Work out the finished part from the listing and answer in its coordinate system (mm). Face numbers are marked on the shaded views. Round coordinates to 2 decimals unless told otherwise and drop trailing zeros. One line per item, written item: value.
```python
from build123d import *

# Parameters (mm, degrees)
CELL_BLOCK_SKETCH_W  = 140.101132068
CELL_BLOCK_SKETCH_H  = 360.075
BOSS_EXTRUDE1_DEPTH  = 5
CELL_HOLES_PATTERN_R = 10.875
CUT_EXTRUDE1_DEPTH   = 5
SKETCH1_R            = 10.875
CUT_EXTRUDE2_DEPTH   = 5
SKETCH3_W            = 15
SKETCH3_H            = 360.075
BOSS_EXTRUDE3_DEPTH  = 10
SKETCH4_R            = 3.25
CUT_EXTRUDE3_DEPTH   = 10


with BuildPart() as part:
    # Cell Block Sketch → Boss-Extrude1 (new body)
    with BuildSketch(Plane(origin=(0, 0, 0), x_dir=(1, 0, 0), z_dir=(0, 1, 0))):
        Rectangle(CELL_BLOCK_SKETCH_W, CELL_BLOCK_SKETCH_H)
    extrude(amount=BOSS_EXTRUDE1_DEPTH)

    # Cell Holes Pattern → Cut-Extrude1 (cut)
    with BuildSketch(Plane(origin=(0, 0, 0), x_dir=(1, 0, 0), z_dir=(0, 1, 0))):
        with Locations(Location((-34.400283017, 137.7875, 0), (0, 0, 270))):
            Circle(CELL_HOLES_PATTERN_R)
        with Locations(Location((-54.275566034, 149.2625, 0), (0, 0, 270))):
            Circle(CELL_HOLES_PATTERN_R)
        with Locations(Location((-14.525, 149.2625, 0), (0, 0, 270))):
            Circle(CELL_HOLES_PATTERN_R)
        with Locations(Location((-54.275566034, 126.3125, 0), (0, 0, 270))):
            Circle(CELL_HOLES_PATTERN_R)
        with Locations(Location((-34.400283017, 114.8375, 0), (0, 0, 270))):
            Circle(CELL_HOLES_PATTERN_R)
        with Locations(Location((-14.525, 126.3125, 0), (0, 0, 270))):
            Circle(CELL_HOLES_PATTERN_R)
        with Locations(Location((-54.275566034, 103.3625, 0), (0, 0, 270))):
            Circle(CELL_HOLES_PATTERN_R)
        with Locations(Location((-34.400283017, 91.8875, 0), (0, 0, 270))):
            Circle(CELL_HOLES_PATTERN_R)
        with Locations(Location((-14.525, 103.3625, 0), (0, 0, 270))):
            Circle(CELL_HOLES_PATTERN_R)
        with Locations(Location((-54.275566034, 80.4125, 0), (0, 0, 270))):
            Circle(CELL_HOLES_PATTERN_R)
        with Locations(Location((-34.400283017, 68.9375, 0), (0, 0, 270))):
            Circle(CELL_HOLES_PATTERN_R)
        with Locations(Location((-14.525, 80.4125, 0), (0, 0, 270))):
            Circle(CELL_HOLES_PATTERN_R)
        with Locations(Location((-54.275566034, 57.4625, 0), (0, 0, 270))):
            Circle(CELL_HOLES_PATTERN_R)
        with Locations(Location((-34.400283017, 45.9875, 0), (0, 0, 270))):
            Circle(CELL_HOLES_PATTERN_R)
        with Locations(Location((-14.525, 57.4625, 0), (0, 0, 270))):
            Circle(CELL_HOLES_PATTERN_R)
        with Locations(Location((-54.275566034, 34.5125, 0), (0, 0, 270))):
            Circle(CELL_HOLES_PATTERN_R)
        with Locations(Location((-34.400283017, 23.0375, 0), (0, 0, 270))):
            Circle(CELL_HOLES_PATTERN_R)
        with Locations(Location((-14.525, 34.5125, 0), (0, 0, 270))):
            Circle(CELL_HOLES_PATTERN_R)
        with Locations(Location((-54.275566034, 11.5625, 0), (0, 0, 270))):
            Circle(CELL_HOLES_PATTERN_R)
        with Locations(Location((-34.400283017, 0.0875, 0), (0, 0, 270))):
            Circle(CELL_HOLES_PATTERN_R)
        with Locations(Location((-14.525, 11.5625, 0), (0, 0, 270))):
            Circle(CELL_HOLES_PATTERN_R)
        with Locations(Location((-54.275566034, -11.3875, 0), (0, 0, 270))):
            Circle(CELL_HOLES_PATTERN_R)
        with Locations(Location((-34.400283017, -22.8625, 0), (0, 0, 270))):
            Circle(CELL_HOLES_PATTERN_R)
        with Locations(Location((-14.525, -11.3875, 0), (0, 0, 270))):
            Circle(CELL_HOLES_PATTERN_R)
        with Locations(Location((-54.275566034, -34.3375, 0), (0, 0, 270))):
            Circle(CELL_HOLES_PATTERN_R)
        with Locations(Location((-34.400283017, -45.8125, 0), (0, 0, 270))):
            Circle(CELL_HOLES_PATTERN_R)
        with Locations(Location((-14.525, -34.3375, 0), (0, 0, 270))):
            Circle(CELL_HOLES_PATTERN_R)
        with Locations(Location((-54.275566034, -57.2875, 0), (0, 0, 270))):
            Circle(CELL_HOLES_PATTERN_R)
        with Locations(Location((-34.400283017, -68.7625, 0), (0, 0, 270))):
            Circle(CELL_HOLES_PATTERN_R)
        with Locations(Location((-14.525, -57.2875, 0), (0, 0, 270))):
            Circle(CELL_HOLES_PATTERN_R)
        with Locations(Location((-54.275566034, -80.2375, 0), (0, 0, 270))):
            Circle(CELL_HOLES_PATTERN_R)
        with Locations(Location((-34.400283017, -91.7125, 0), (0, 0, 270))):
            Circle(CELL_HOLES_PATTERN_R)
        with Locations(Location((-14.525, -80.2375, 0), (0, 0, 270))):
            Circle(CELL_HOLES_PATTERN_R)
        with Locations(Location((-54.275566034, -103.1875, 0), (0, 0, 270))):
            Circle(CELL_HOLES_PATTERN_R)
        with Locations(Location((-34.400283017, -114.6625, 0), (0, 0, 270))):
            Circle(CELL_HOLES_PATTERN_R)
        with Locations(Location((-14.525, -103.1875, 0), (0, 0, 270))):
            Circle(CELL_HOLES_PATTERN_R)
        with Locations(Location((-54.275566034, -126.1375, 0), (0, 0, 270))):
            Circle(CELL_HOLES_PATTERN_R)
        with Locations(Location((-34.400283017, -137.6125, 0), (0, 0, 270))):
            Circle(CELL_HOLES_PATTERN_R)
        with Locations(Location((-14.525, -126.1375, 0), (0, 0, 270))):
            Circle(CELL_HOLES_PATTERN_R)
        with Locations(Location((-54.275566034, -149.0875, 0), (0, 0, 270))):
            Circle(CELL_HOLES_PATTERN_R)
        with Locations(Location((-34.400283017, -160.5625, 0), (0, 0, 270))):
            Circle(CELL_HOLES_PATTERN_R)
        with Locations(Location((-14.525, -149.0875, 0), (0, 0, 270))):
            Circle(CELL_HOLES_PATTERN_R)
    extrude(amount=CUT_EXTRUDE1_DEPTH, mode=Mode.SUBTRACT)

    # Sketch1 → Cut-Extrude2 (cut)
    with BuildSketch(Plane(origin=(0, 5, 0), x_dir=(1, 0, 0), z_dir=(0, 1, 0))):
        with Locations(Location((14.525, 137.7875, 0), (0, 0, 270))):
            Circle(SKETCH1_R)
        with Locations(Location((34.400283017, 149.2625, 0), (0, 0, 270))):
            Circle(SKETCH1_R)
        with Locations(Location((54.275566034, 137.7875, 0), (0, 0, 270))):
            Circle(SKETCH1_R)
        with Locations(Location((14.525, 114.8375, 0), (0, 0, 270))):
            Circle(SKETCH1_R)
        with Locations(Location((34.400283017, 126.3125, 0), (0, 0, 270))):
            Circle(SKETCH1_R)
        with Locations(Location((54.275566034, 114.8375, 0), (0, 0, 270))):
            Circle(SKETCH1_R)
        with Locations(Location((14.525, 91.8875, 0), (0, 0, 270))):
            Circle(SKETCH1_R)
        with Locations(Location((34.400283017, 103.3625, 0), (0, 0, 270))):
            Circle(SKETCH1_R)
        with Locations(Location((54.275566034, 91.8875, 0), (0, 0, 270))):
            Circle(SKETCH1_R)
        with Locations(Location((14.525, 68.9375, 0), (0, 0, 270))):
            Circle(SKETCH1_R)
        with Locations(Location((34.400283017, 80.4125, 0), (0, 0, 270))):
            Circle(SKETCH1_R)
        with Locations(Location((54.275566034, 68.9375, 0), (0, 0, 270))):
            Circle(SKETCH1_R)
        with Locations(Location((14.525, 45.9875, 0), (0, 0, 270))):
            Circle(SKETCH1_R)
        with Locations(Location((34.400283017, 57.4625, 0), (0, 0, 270))):
            Circle(SKETCH1_R)
        with Locations(Location((54.275566034, 45.9875, 0), (0, 0, 270))):
            Circle(SKETCH1_R)
        with Locations(Location((14.525, 23.0375, 0), (0, 0, 270))):
            Circle(SKETCH1_R)
        with Locations(Location((34.400283017, 34.5125, 0), (0, 0, 270))):
            Circle(SKETCH1_R)
        with Locations(Location((54.275566034, 23.0375, 0), (0, 0, 270))):
            Circle(SKETCH1_R)
        with Locations(Location((14.525, 0.0875, 0), (0, 0, 270))):
            Circle(SKETCH1_R)
        with Locations(Location((34.400283017, 11.5625, 0), (0, 0, 270))):
            Circle(SKETCH1_R)
        with Locations(Location((54.275566034, 0.0875, 0), (0, 0, 270))):
            Circle(SKETCH1_R)
        with Locations(Location((14.525, -22.8625, 0), (0, 0, 270))):
            Circle(SKETCH1_R)
        with Locations(Location((34.400283017, -11.3875, 0), (0, 0, 270))):
            Circle(SKETCH1_R)
        with Locations(Location((54.275566034, -22.8625, 0), (0, 0, 270))):
            Circle(SKETCH1_R)
        with Locations(Location((14.525, -45.8125, 0), (0, 0, 270))):
            Circle(SKETCH1_R)
        with Locations(Location((34.400283017, -34.3375, 0), (0, 0, 270))):
            Circle(SKETCH1_R)
        with Locations(Location((54.275566034, -45.8125, 0), (0, 0, 270))):
            Circle(SKETCH1_R)
        with Locations(Location((14.525, -68.7625, 0), (0, 0, 270))):
            Circle(SKETCH1_R)
        with Locations(Location((34.400283017, -57.2875, 0), (0, 0, 270))):
            Circle(SKETCH1_R)
        with Locations(Location((54.275566034, -68.7625, 0), (0, 0, 270))):
            Circle(SKETCH1_R)
        with Locations(Location((14.525, -91.7125, 0), (0, 0, 270))):
            Circle(SKETCH1_R)
        with Locations(Location((34.400283017, -80.2375, 0), (0, 0, 270))):
            Circle(SKETCH1_R)
        with Locations(Location((54.275566034, -91.7125, 0), (0, 0, 270))):
            Circle(SKETCH1_R)
        with Locations(Location((14.525, -114.6625, 0), (0, 0, 270))):
            Circle(SKETCH1_R)
        with Locations(Location((34.400283017, -103.1875, 0), (0, 0, 270))):
            Circle(SKETCH1_R)
        with Locations(Location((54.275566034, -114.6625, 0), (0, 0, 270))):
            Circle(SKETCH1_R)
        with Locations(Location((14.525, -137.6125, 0), (0, 0, 270))):
            Circle(SKETCH1_R)
        with Locations(Location((34.400283017, -126.1375, 0), (0, 0, 270))):
            Circle(SKETCH1_R)
        with Locations(Location((54.275566034, -137.6125, 0), (0, 0, 270))):
            Circle(SKETCH1_R)
        with Locations(Location((14.525, -160.5625, 0), (0, 0, 270))):
            Circle(SKETCH1_R)
        with Locations(Location((34.400283017, -149.0875, 0), (0, 0, 270))):
            Circle(SKETCH1_R)
        with Locations(Location((54.275566034, -160.5625, 0), (0, 0, 270))):
            Circle(SKETCH1_R)
    extrude(amount=-CUT_EXTRUDE2_DEPTH, mode=Mode.SUBTRACT)

    # Sketch3 → Boss-Extrude3 (add)
    with BuildSketch(Plane(origin=(0, 0, 0), x_dir=(1, 0, 0), z_dir=(0, 1, 0))):
        with Locations((-77.550566034, 0)):
            Rectangle(SKETCH3_W, SKETCH3_H)
    boss_extrude3 = extrude(amount=BOSS_EXTRUDE3_DEPTH)

    # Mirror1: Boss-Extrude3 across plane
    add(boss_extrude3.mirror(Plane(origin=(0, 0, 0), x_dir=(0, 0, 1), z_dir=(1, 0, 0))))

    # Sketch4 → Cut-Extrude3 (cut)
    with BuildSketch(Plane(origin=(0, 10, 0), x_dir=(1, 0, 0), z_dir=(0, 1, 0))):
        with Locations(Location((-77.550566034, 0, 0), (0, 0, 270))):
            Circle(SKETCH4_R)
        with Locations(Location((-77.550566034, -50, 0), (0, 0, 270))):
            Circle(SKETCH4_R)
        with Locations(Location((-77.550566034, -100, 0), (0, 0, 270))):
            Circle(SKETCH4_R)
        with Locations(Location((-77.550566034, 50, 0), (0, 0, 270))):
            Circle(SKETCH4_R)
        with Locations(Location((-77.550566034, 100, 0), (0, 0, 270))):
            Circle(SKETCH4_R)
    cut_extrude3 = extrude(amount=-CUT_EXTRUDE3_DEPTH, mode=Mode.SUBTRACT)

    # Mirror2: Cut-Extrude3 across plane
    add(cut_extrude3.mirror(Plane(origin=(0, 0, 0), x_dir=(0, 0, 1), z_dir=(1, 0, 0))), mode=Mode.SUBTRACT)


solid = part.part
```
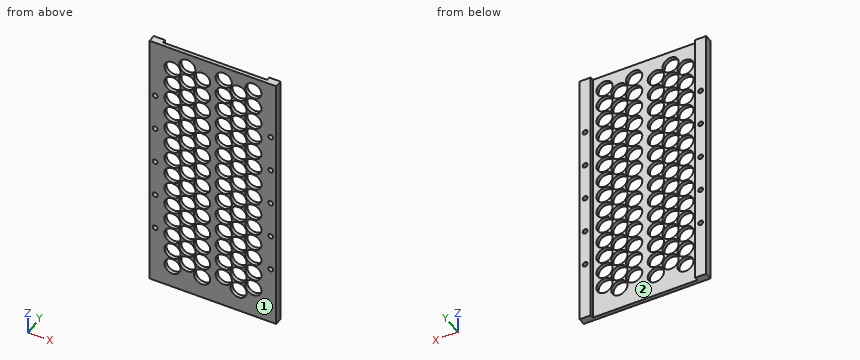
(1) Find section A-A on z = -30.5. Give the number of separate pieces and of enclosed holes in the cut face, plus the area to 3 significant figures.
Reported:
separate pieces: 7
enclosed holes: 0
area: 460 mm2
(2) A flat-ended cylindrical pin translates along its axis: pin 1 Ø25 at (x, z) = (54.28, 91.71) entering from +Y. Find the tip coordinate at first contact, or state that the pin passes through.
Reported:
pin 1: stops at y = 5
(3) For a pull along X with two mould halves and no side action, classify the marked faces 1 and 2 as pulls with the +X half, pulls with the -X half, needs draft (parallel to the pull), parting line crosses it, or undercut.
Reported:
face 1: needs draft
face 2: undercut
(4) Consider probe 1 along X at (y, z) = (6, -59); probe 2 along Z at (x, y) = (-75, 9); probe 3 along Y at (x, z) = (67, -129.5). Determine where each line is inside the solid, lowest interval first.
Reported:
probe 1: x = -85.05 to -70.05, 70.05 to 85.05
probe 2: z = -180.04 to -102.01, -97.99 to -52.01, -47.99 to -2.01, 2.01 to 47.99, 52.01 to 97.99, 102.01 to 180.04
probe 3: y = 0 to 5
